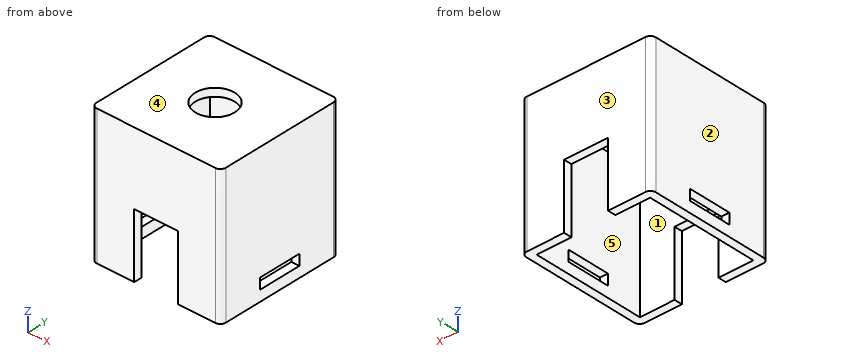
Autodesk Inventor part; units mm, degrees
ref_plane "YZ Plane" through (0, 0, 0) normal (1, 0, 0) x (0, 1, 0)
ref_plane "XZ Plane" through (0, 0, 0) normal (0, 1, 0) x (-1, 0, 0)
ref_plane "XY Plane" through (0, 0, 0) normal (0, 0, 1) x (1, 0, 0)
sketch "Sketch1" plane through (0, 0, 0) normal (0, 0, 1) x (1, 0, 0)
  line L0 (0, 0) -> (76.2, 0)
  line L1 (76.2, 0) -> (76.2, 76.2)
  line L2 (76.2, 76.2) -> (0, 76.2)
  line L3 (0, 76.2) -> (0, 0)
  dimension "d0" = 76.2
  dimension "d1" = 76.2
extrude "Extrusion1" add sketch "Sketch1" along normal blind 4.699
sketch "Sketch2" plane through (0, 0, 4.699) normal (0, 0, 1) x (1, 0, 0)
  point P0 (0, 0)
sketch "Sketch3" plane through (0, 0, 4.699) normal (0, 0, 1) x (1, 0, 0)
  circle A0 centre (38.1, 38.1) radius 11.6205
  line L0 (0, 76.2) -> (0, 0)
  line L1 (0, 0) -> (76.2, 0)
  point P0 (0, 73.025)
  point P1 (0, 3.175)
  point P2 (3.175, 0)
  point P3 (73.025, 0)
  dimension "d5" = 23.241
  dimension "d6" = 38.1
  dimension "d7" = 38.1
extrude "Extrusion2" cut sketch "Sketch3" against normal blind 4.699
sketch "Sketch5" plane through (0, 0, 0) normal (0, 0, -1) x (-1, 0, 0)
  line L0 (-4.699, 4.699) -> (-71.501, 4.699)
  line L1 (-71.501, 4.699) -> (-71.501, 71.501)
  line L2 (-71.501, 71.501) -> (-4.699, 71.501)
  line L3 (-4.699, 71.501) -> (-4.699, 4.699)
  line L4 (0, 0) -> (-76.2, 0)
  line L5 (0, 76.2) -> (0, 0)
  line L6 (-76.2, 76.2) -> (0, 76.2)
  line L7 (-76.2, 0) -> (-76.2, 76.2)
  line L8 (0, 76.2) -> (0, 0)
  line L9 (0, 0) -> (-76.2, 0)
  line L10 (-76.2, 0) -> (-76.2, 76.2)
  line L11 (-76.2, 76.2) -> (0, 76.2)
  line L12 (0, 76.2) -> (0, 0)
  dimension "d18" = 4.699
  dimension "d19" = 4.699
  dimension "d20" = 4.699
  dimension "d21" = 4.699
extrude "Extrusion4" add sketch "Sketch5" along normal blind 76.2
sketch "Sketch6" plane through (0, 0, 4.699) normal (0, -1, 0) x (1, 0, 0)
  line L0 (4.699, -80.899) -> (71.501, -80.899)
  line L1 (25.146, -80.899) -> (51.054, -80.899)
  line L2 (51.054, -80.899) -> (51.054, -42.7482)
  line L3 (51.054, -42.7482) -> (25.146, -42.7482)
  line L4 (25.146, -42.7482) -> (25.146, -80.899)
  line L5 (76.2, -80.899) -> (76.2, 0)
  line L6 (0, 0) -> (0, -80.899)
  point P0 (0, -4.699)
  dimension "d24" = 25.908
  dimension "d25" = 38.1508
  dimension "d26" = 25.146
  dimension "d27" = 25.146
extrude "Extrusion5" cut sketch "Sketch6" against normal through all
sketch "Sketch7" plane through (76.2, 0, 4.699) normal (1, 0, 0) x (0, 0, -1)
  line L0 (74.549, 25.4) -> (68.199, 25.4)
  line L1 (68.199, 25.4) -> (68.199, 50.8)
  line L2 (68.199, 50.8) -> (74.549, 50.8)
  line L3 (74.549, 50.8) -> (74.549, 25.4)
  line L4 (80.899, 76.2) -> (80.899, 0)
  line L5 (80.899, 76.2) -> (0, 76.2)
  line L6 (80.899, 0) -> (0, 0)
  point P0 (4.699, 0)
  dimension "d30" = 6.35
  dimension "d31" = 25.4
  dimension "d32" = 6.35
  dimension "d33" = 25.4
  dimension "d34" = 25.4
extrude "Extrusion6" cut sketch "Sketch7" against normal through all
fillet "Fillet2" radius 3.175 4 edges at (76.2, 76.2, -35.7505) (0, 76.2, -35.7505) (76.2, 0, -35.7505) (0, 0, -35.7505)
properties part number "buttonInchPipeMount"
Verification items for the finished model (mm, model axes). Face numbers are marked on the shaded views. A direction names the side the tool comes from. Round coordinates to 2 decimals unless told otherwise and drop trailing zeros. Order: outer loops, then holes, each group sorted by start corner. A loop starts at its lowest first (then second) coordinate and runs counter-clockwise, first axis right, second up.
1) Cross-section at D-D, the plane z = -3.5. Record the cut outline in (x, y) (3 decimals).
Geometry says:
outline: (0, 3.175) arc R3.175 ccw to (3.175, 0) - (73.025, 0) arc R3.175 ccw to (76.2, 3.175) - (76.2, 73.025) arc R3.175 ccw to (73.025, 76.2) - (3.175, 76.2) arc R3.175 ccw to (0, 73.025) - close; hole (4.699, 4.699) - (71.501, 4.699) - (71.501, 71.501) - (4.699, 71.501) - close
2) Material ranges on line 1 (X direction, y = 38, z = 3); line 2 (X direction, y = 29.5, z = -1), recorded low to high.
Geometry says:
line 1: x = 0 to 26.48, 49.72 to 76.2
line 2: x = 0 to 4.7, 71.5 to 76.2
3) Tool access check on the marked faces 4 and 5. Record the directions out of +Z, -Z, +X, -X, +Y, -Y that give a thin tool (end or side, any length) a straight path to the whole face; none if there is none.
Geometry says:
face 4: +Z, +X, -X, +Y, -Y
face 5: -Z
4) Cross-section at B-B, the plane y = 38.1. Record the cut outline in (x, z).
Geometry says:
outline: (0, -76.2) - (4.7, -76.2) - (4.7, -69.85) - (0, -69.85) - close; (0, -63.5) - (4.7, -63.5) - (4.7, 0) - (26.48, 0) - (26.48, 4.7) - (0, 4.7) - close; (49.72, 0) - (71.5, 0) - (71.5, -63.5) - (76.2, -63.5) - (76.2, 4.7) - (49.72, 4.7) - close; (71.5, -76.2) - (76.2, -76.2) - (76.2, -69.85) - (71.5, -69.85) - close
5) Cross-section at C-C, the plane x = 38.1. Record the cut outline in (y, z), plus the area to 3 significant figures.
Geometry says:
outline: (0, -38.05) - (4.7, -38.05) - (4.7, 0) - (26.48, 0) - (26.48, 4.7) - (0, 4.7) - close; (49.72, 0) - (71.5, 0) - (71.5, -38.05) - (76.2, -38.05) - (76.2, 4.7) - (49.72, 4.7) - close
area: 606 mm2
6) Cross-section at A-A, the plane z = -55. Record the cut outline in (x, y) (3 decimals).
Geometry says:
outline: (0, 3.175) arc R3.175 ccw to (3.175, 0) - (25.146, 0) - (25.146, 4.699) - (4.699, 4.699) - (4.699, 71.501) - (25.146, 71.501) - (25.146, 76.2) - (3.175, 76.2) arc R3.175 ccw to (0, 73.025) - close; (51.054, 0) - (73.025, 0) arc R3.175 ccw to (76.2, 3.175) - (76.2, 73.025) arc R3.175 ccw to (73.025, 76.2) - (51.054, 76.2) - (51.054, 71.501) - (71.501, 71.501) - (71.501, 4.699) - (51.054, 4.699) - close
7) Draft check along Y on the marked faces 1, 2 and 3. Enter one of: +Y half, -Y half, draft (parallel to the pull), parting line (faces both ways), or undercut.
Geometry says:
face 1: undercut
face 2: draft
face 3: +Y half
8) Depth check by flat-ended pin: pin 1 (1.4 mm diameter, centred on x = 74, z = -67, fed in from -Y); pin 2 (2.5 mm diameter, centred on x = 35.5, y = 72.5, fed in from -Z); pin 3 (20 mm diameter, centred on x = 39, y = 24, fed in from -Z); pin 4 (14 mm diameter, centred on x = 38.1, y = 38.1, fed in from -Z). Enter the tip coordinate at first touch or a pass-through.
Geometry says:
pin 1: stops at y = 0.01
pin 2: stops at z = -38.05
pin 3: stops at z = 0
pin 4: passes through
